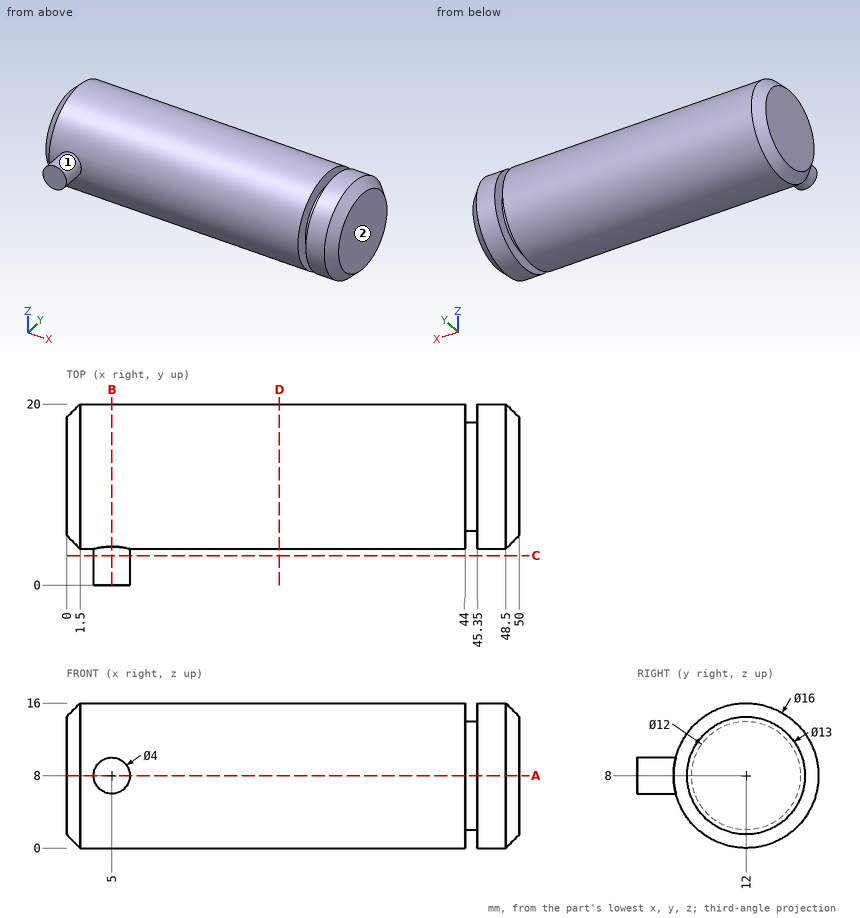
Can you work these out from the drawing? Everything is in mm from the part's minimum corner. A direction names the side the tool comes from. Round coordinates to 2 decimals unless told otherwise and drop trailing zeros. Order: outer loops, then holes, each group sorted by start corner. A loop starts at its lowest first (then second) coordinate and runs counter-clockwise, first axis right, second up.
(1) On a 3-axis mill with a long thin cutter (end or side, diameter ignored), from which of +Z, -Z, +X, -X, +Y, -Y can I reach the whole of each face in a straight line? I mean the marked faces 1 and 2. Say none if no direction works.
Results are:
face 1: -Y
face 2: +Z, -Z, +X, +Y, -Y
(2) If we section it at C-C (y = 3.25): Please give me the cut outline in (x, z).
Results are:
outline: circle Ø4 at (5, 8)
(3) If we section it at B-B (x = 5): Please give me the cut outline in (y, z), plus the area to 3 significant figures.
Results are:
outline: (0, 6) - (4.25, 6) arc R8 ccw (long way) to (4.25, 10) - (0, 10) - close
area: 217 mm2
(4) If we section it at D-D (x = 23.5): Please give me the cut outline in (y, z), plus the area to 3 significant figures.
Results are:
outline: circle Ø16 at (12, 8)
area: 201 mm2
(5) If we section it at A-A (z = 8): Please give me the cut outline in (x, y), plus the area to 3 significant figures.
Results are:
outline: (0, 5.5) - (1.5, 4) - (3, 4) - (3, 0) - (7, 0) - (7, 4) - (44, 4) - (44, 6) - (45.35, 6) - (45.35, 4) - (48.5, 4) - (50, 5.5) - (50, 18.5) - (48.5, 20) - (45.35, 20) - (45.35, 18) - (44, 18) - (44, 20) - (1.5, 20) - (0, 18.5) - close
area: 806 mm2
(6) If I drill on L1, parallel to Z at x = 14.5, y = 11.75; L2, parallel to X at y = 18, z = 11; L3, parallel to X at y = 4.75, z = 8.5, over which ranges is the centre line in solid material (lowest first)?
Results are:
L1: z = 0 to 16
L2: x = 0.21 to 44, 45.35 to 49.79
L3: x = 0.77 to 44, 45.35 to 49.23
(7) I'm going to push flat-ended pins straight in: pin 1 (5 mm diameter, centred on x = 20, y = 3.5, fed in from -Z); pin 2 (12 mm diameter, centred on x = 20.5, y = 2.5, fed in from -Z); pin 3 (1 mm diameter, centred on x = 33.5, y = 10.5, fed in from -Z). Where does each tip first touch, or does it pass through?
Results are:
pin 1: stops at z = 2.71
pin 2: stops at z = 0.81
pin 3: stops at z = 0.06
